Part model, mm, in its own coordinate system. Face numbers are marked on the shaded views. A direction names the side the tool comes from. Round coordinates to 2 decimals unless told otherwise and drop trailing zeros. Write each loop counter-clockwise with the first axis right and the second up, starting at its lowest first coordinate (ties: lowest second). Pieces come first, ordered by that corner, then holes.
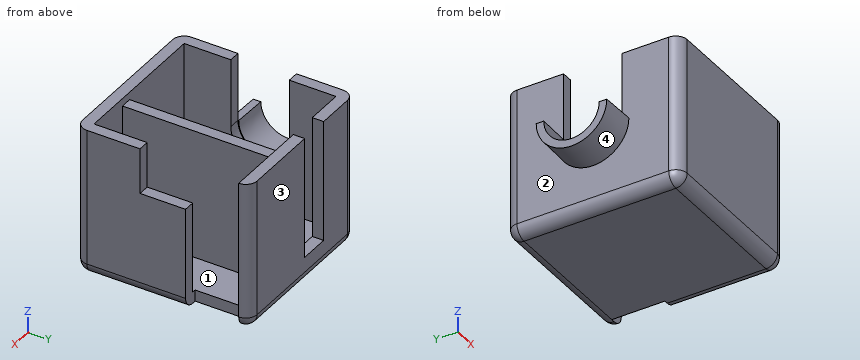
```python
from build123d import *

# Parameters (mm, degrees)
CONE_ANGLE      = 180
THICKNESS001_T  = 1
BOX_W           = 19
BOX_H           = 20
BOX_DEPTH       = 18
THICKNESS_T     = 1.5
POCKET_DEPTH    = 2
SKETCH001_W     = 4
SKETCH001_H     = 18
POCKET001_DEPTH = 2
BOX001_W        = 20
BOX001_H        = 17
BOX001_DEPTH    = 1.5
POCKET002_DEPTH = 2


with BuildPart() as thickness001:
    # Cone → Cone (revolve)
    with BuildSketch(Plane(origin=(-1.5, 10, 9), x_dir=(0, 1, 0), z_dir=(0, 0, 1))):
        Polygon((0, 0), (3.75, 0), (3.65, 4.5), (0, 4.5), align=None)
    revolve(axis=Axis((-1.5, 10, 9), (-1, 0, 0)), revolution_arc=CONE_ANGLE)

    # Thickness001
    thickness001_openings = [thickness001.faces().sort_by_distance(p)[0] for p in [
        (-3.739865, 8.149887, 9),
        (-3.739865, 11.850113, 9),
        (-6, 10, 7.450892),
        (-1.5, 10, 7.408451),
    ]]
    offset(amount=THICKNESS001_T, openings=thickness001_openings)


with BuildPart() as fusion:
    # Box → Box (join)
    with BuildSketch(Plane.XY):
        with Locations((9.5, 10)):
            Rectangle(BOX_W, BOX_H)
    extrude(amount=BOX_DEPTH)

    # Thickness
    thickness_openings = [fusion.faces().sort_by_distance(p)[0] for p in [
        (9.5, 10, 18),
    ]]
    offset(amount=THICKNESS_T, openings=thickness_openings)

    # Sketch (on Face7 of Thickness) → Pocket (cut)
    with BuildSketch(Plane(origin=(-1.5, 0, 0), x_dir=(0, -1, 0), z_dir=(-1, 0, 0))):
        with BuildLine():
            ThreePointArc((-6.15, 19), (-10, 22.85), (-13.85, 19))
            Line((-13.85, 19), (-13.85, 9))
            ThreePointArc((-13.85, 9), (-10, 5.15), (-6.15, 9))
            Line((-6.15, 19), (-6.15, 9))
        make_face()
    extrude(amount=-POCKET_DEPTH, mode=Mode.SUBTRACT)

    # Sketch001 (on Face10 of Pocket) → Pocket001 (cut)
    with BuildSketch(Plane(origin=(0, 21.5, 0), x_dir=(-1, 0, 0), z_dir=(0, 1, 0))):
        with Locations((-7, 11)):
            Rectangle(SKETCH001_W, SKETCH001_H)
    extrude(amount=-POCKET001_DEPTH, mode=Mode.SUBTRACT)

    # Box001 → Box001 (join)
    with BuildSketch(Plane.YZ.offset(11.5)):
        with Locations((10, 8.5)):
            Rectangle(BOX001_W, BOX001_H)
    extrude(amount=BOX001_DEPTH)

    # Sketch002 (on Face14 of Box001) → Pocket002 (cut)
    with BuildSketch(Plane.YZ.offset(20.5)):
        Polygon((20, 18), (7, 18), (7, 12), (13, 12), (13, -10.564874), (20, -10.564874), align=None)
    extrude(amount=-POCKET002_DEPTH, mode=Mode.SUBTRACT)

    # Fusion: union Thickness001
    add(thickness001.part)


solid = fusion.part
```
Q1. Wall check: L1, parallel to X at y = 5.75, z = 0.5; L2, parallel to X at y = 6.5, z = 6.5; L3, parallel to Y at x = 11.25, z = 15. Give the ranges that are in metal, low to high.
Values follow:
L1: x = -1.5 to 0, 11.5 to 13, 19 to 20.5
L2: x = -6 to 0, 11.5 to 13, 19 to 20.5
L3: y = -1.5 to 0, 20 to 21.5
Q2. Which spindle directions (+Z, -Z, +X, -X, +Y, -Y) get a long thin tool onto all of the face, cutting with end or side? Do the marked faces 1, 2, 3 and 4. Say none if no direction does.
Values follow:
face 1: +Z
face 2: -X
face 3: +Z, -Z, +X, -X, +Y
face 4: -Z, -X
Q3. Drop flat-ended pins along their axis: pin 1 (5 mm diameter, centred on x = 15, y = 14.5, fed in from +Z); pin 2 (1.6 mm diameter, centred on y = 16, z = -0.5, fed in from +X); pin 3 (1.2 mm diameter, centred on x = -1, z = 11.5, fed in from +Y). Give the stop position or say it passes through.
Values follow:
pin 1: stops at z = 17
pin 2: stops at x = 18.5
pin 3: stops at y = 21.45
Q4. Cut at D-D on x = 13.5. Write the cut outline in (y, z), plus the area to 3 significant figures.
Values follow:
outline: (-1.5, 0) arc R1.5 ccw to (0, -1.5) - (20, -1.5) arc R1.5 ccw to (21.5, 0) - (21.5, 18) - (20, 18) - (20, 0) - (0, 0) - (0, 18) - (-1.5, 18) - close
area: 87.5 mm2
Q5. Cut at B-B on z = 1.25. Write the cut outline in (x, y), plus the area to 3 significant figures.
Values follow:
outline: (-1.5, 0) arc R1.5 ccw to (0, -1.5) - (19, -1.5) arc R1.5 ccw to (20.5, 0) - (20.5, 13) - (19, 13) - (19, 0) - (13, 0) - (13, 20) - (20.5, 20) arc R1.5 ccw to (19, 21.5) - (0, 21.5) arc R1.5 ccw to (-1.5, 20) - close; hole (0, 0) - (11.5, 0) - (11.5, 20) - (0, 20) - close
area: 144 mm2
Q6. Cut at C-C on y = 10. Write the cut outline in (x, z), plus the area to 3 significant figures.
Values follow:
outline: (-6, 4.35) - (-1.5, 4.25) - (-1.5, 0) arc R1.5 ccw to (0, -1.5) - (19, -1.5) arc R1.5 ccw to (20.5, 0) - (20.5, 12) - (19, 12) - (19, 0) - (13, 0) - (13, 17) - (11.5, 17) - (11.5, 0) - (0, 0) - (0, 5.15) - (-1.5, 5.15) - (-1.5, 5.25) - (-6, 5.35) - close
area: 87.8 mm2
Q7. Cut at A-A on z = 11. Write the cut outline in (x, y), plus the area to 3 significant figures.
Values follow:
outline: (-1.5, 0) arc R1.5 ccw to (0, -1.5) - (19, -1.5) arc R1.5 ccw to (20.5, 0) - (20.5, 13) - (19, 13) - (19, 0) - (13, 0) - (13, 20) - (20.5, 20) arc R1.5 ccw to (19, 21.5) - (9, 21.5) - (9, 20) - (11.5, 20) - (11.5, 0) - (0, 0) - (0, 6.15) - (-1.5, 6.15) - close; (-1.5, 13.85) - (0, 13.85) - (0, 20) - (5, 20) - (5, 21.5) - (0, 21.5) arc R1.5 ccw to (-1.5, 20) - close
area: 126 mm2
